Here's how the part is built. I have some questions about the finished solid (model axes, mm). A direction names the side the tool comes from. Coordinates: 2 decimals unless noted, no trailing zeros. Write each loop counter-clockwise with the first axis right and the second up, starting at its lowest first coordinate (ties: lowest second). Pieces come first, ordered by that corner, then holes.
Item 1: I'm going to push flat-ended pins straight in: pin 1 Ø2 at (x, y) = (-434, 4) entering from +Z; pin 2 Ø2 at (y, z) = (4.5, 219.5) entering from +X; pin 3 Ø1 at (y, z) = (1, -21.5) entering from +X. Where does each tip first touch, or does it pass through?
Item 2: If we section it at B-B (z = 35.5): Please give me the cut outline in (x, y).
Item 3: If I drill on line 1 (X direction, y = 2.75, z = -40); line 2 (Z direction, x = -436, y = 4.75); line 3 (Z direction, x = -428, y = 0.5), over which ranges is the centre line in solid material (lowest first)?
Item 4: If we section it at C-C (x = -431): Please give me the cut outline in (y, z).
Item 5: If we section it at A-A (y = 3): Please give me the cut outline in (x, z), then the cut area to 3 significant figures.
Item 6: For faces 1 (the face through (-500, 3, -39)), 2 (the face through (-470, 3, -39)), which set-ups out of +Z, -Z, +X, -X, +Y, -Y let a thin tool reach every point of the face, with its end or its side?
from build123d import *

# Parameters (mm, degrees)
BOSS_EXTRUDE1_DEPTH = 6.35
SKETCH3_W           = 30
SKETCH3_H           = 6.35
BOSS_EXTRUDE2_DEPTH = 80


with BuildPart() as part:
    # Sketch2 → Boss-Extrude1 (new body)
    with BuildSketch(Plane(origin=(0, 0, 0), x_dir=(1, 0, 0), z_dir=(0, 1, 0))):
        with BuildLine():
            ThreePointArc((0, -470), (-332.340187158, -332.340187158), (-470, 0))
            Line((-470, 0), (-500, 0))
            ThreePointArc((-500, 0), (-353.553390593, -353.553390593), (0, -500))
            Line((0, -500), (0, -470))
        make_face()
    extrude(amount=BOSS_EXTRUDE1_DEPTH)

    # Sketch3 → Boss-Extrude2 (add)
    with BuildSketch(Plane(origin=(0, 0, 0), x_dir=(-1, 0, 0), z_dir=(0, 0, -1))):
        with Locations((485, 3.175)):
            Rectangle(SKETCH3_W, SKETCH3_H)
    extrude(amount=BOSS_EXTRUDE2_DEPTH)

    # Split1
    split(bisect_by=Plane(origin=(0, 0, 301), x_dir=(-1, 0, 0), z_dir=(0, 0, -1)), keep=Keep.TOP)


solid = part.part
Answer list:
1. pin 1: stops at z = 250.02
1. pin 2: stops at x = -415.07
1. pin 3: stops at x = -470
2. outline: (-498.74, 0) - (-468.66, 0) - (-468.66, 6.35) - (-498.74, 6.35) - close
3. line 1: x = -500 to -470
3. line 2: z = 175.51 to 244.75
3. line 3: z = 194.21 to 258.49
4. outline: (0, 187.45) - (6.35, 187.45) - (6.35, 253.45) - (0, 253.45) - close
5. outline: (-500, -80) - (-470, -80) - (-470, 0) arc R470 cw to (-360.97, 301) - (-399.25, 301) arc R500 ccw to (-500, 0) - close
5. area: 12,100 mm2
6. face 1: +Z, -Z, -X, +Y, -Y
6. face 2: -Z, +X, +Y, -Y
